Model file for the job. Use its own axes, mm. Coordinates: 2 decimals unless noted, no trailing zeros. Write each loop counter-clockwise with the first axis right and the second up, starting at its lowest first coordinate (ties: lowest second). Pieces come first, ordered by that corner, then holes. Notation, with made-up numbers: (62, 26.25) -> (85, 26.25) arc R10 ccw to (85, 44.25) -> close; hole circle Ø4 at (68.5, -35). An arc over 180 degrees is marked (long way). Answer as a JSON object with one key per item and string values. Group by question number.
Autodesk Inventor part; units mm, degrees
ref_plane "YZ Plane" through (0, 0, 0) normal (1, 0, 0) x (0, 1, 0)
ref_plane "XZ Plane" through (0, 0, 0) normal (0, 1, 0) x (-1, 0, 0)
ref_plane "XY Plane" through (0, 0, 0) normal (0, 0, 1) x (1, 0, 0)
sketch "main" plane through (0, 0, 0) normal (0, 0, 1) x (1, 0, 0)
  circle A0 centre (4.313, -2.5933) radius 2.0828
  circle A1 centre (17.2471, 11.4133) radius 2.1844
  circle A2 centre (-8.1529, 11.4133) radius 2.1844
  arc A3 (-8.1529, 16.1758) -> (-11.7104, 8.2471) centre (-8.1529, 11.4133) ccw
  arc A4 (20.746, 8.1824) -> (17.2471, 16.1758) centre (17.2471, 11.4133) ccw
  arc A5 (0.7554, -5.7596) -> (7.8119, -5.8243) centre (4.313, -2.5933) ccw
  line L0 (20.746, 8.1824) -> (7.8119, -5.8243)
  line L1 (17.2471, 16.1758) -> (-8.1529, 16.1758)
  line L2 (-11.7104, 8.2471) -> (0.7554, -5.7596)
  point P0 (4.4691, 6.7444)
  dimension "d0" = 4.1656
  dimension "d1" = 9.525
  dimension "d2" = 9.525
  dimension "d3" = 9.525
sketch "Sketch1" plane through (0, 0, 0) normal (0, 0, 1) x (1, 0, 0)
  circle A0 centre (-12.5245, 13.9543) radius 2.0828
  circle A1 centre (-25.3998, -0.1065) radius 2.1844
  circle A2 centre (0, 0) radius 2.1844
  arc A3 (0.02, -4.7625) -> (3.5443, 3.1811) centre (0, 0) ccw
  arc A4 (-28.9122, 3.1098) -> (-25.3798, -4.8689) centre (-25.3998, -0.1065) ccw
  arc A5 (-8.9802, 17.1354) -> (-16.0369, 17.1706) centre (-12.5245, 13.9543) ccw
  line L0 (-28.9122, 3.1098) -> (-16.0369, 17.1706)
  line L1 (-25.3798, -4.8689) -> (0.02, -4.7625)
  line L2 (3.5443, 3.1811) -> (-8.9802, 17.1354)
  point P0 (0, 0)
extrude "Extrusion1" add sketch "Sketch1" along normal blind 1.5875
properties part number "brace_gusset" material "Acetal Resin, White"
(1) Wall check: probe 1 along Y at (x, z) = (1, 0.5); probe 2 along X at (y, z) = (15.25, 0.75); probe 3 along Y at (x, z) = (-12, 0.85). Give the ranges that are in metal, low to high.
(2) Cut at A-A on x = -27. List the corners of the cut face in (y, z).
(3) Cut at B-B on y = 14.75. List the corners of the cut face in (x, z), plus the area to 3 significant figures.
(4) Cut at D-D on y = 8.5. List the corners of the cut face in (x, z).
(5) Cut at C-C on z = 0.7. List the corners of the cut face in (x, y), plus the area to 3 significant figures.
(6) Pin check, flat tips, straight feed: pin 1 (2.5 mm diameter, centred on x = -25.4, y = -0.11, fed in from +Z); pin 2 (10 mm diameter, centred on x = -21, y = 13.5, fed in from +Z). Stop position of each tip, or through.
(7) Pull direction X, two halves, no side cores. Call faces 1 (the face through (-12.556, 18.717, 0.783)), 2 (the face through (-27.133, 1.223, 0.783)), 3 (the face through (-13, 4, 0)): released by +X, released by -X, zero draft, split by the parting line, or undercut.
Results found:
{
 "1": {"probe 1": "y = -4.66 to -1.94, 1.94 to 6.02", "probe 2": "x = -17.8 to -14.16, -10.89 to -7.29", "probe 3": "y = -4.81 to 11.94, 15.97 to 18.69"},
 "2": {"outline": "(-4.59, 0) -> (-1.59, 0) -> (-1.59, 1.59) -> (-4.59, 1.59) -> close; (1.38, 0) -> (5.2, 0) -> (5.2, 1.59) -> (1.38, 1.59) -> close"},
 "3": {"outline": "(-18.25, 0) -> (-14.45, 0) -> (-14.45, 1.59) -> (-18.25, 1.59) -> close; (-10.6, 0) -> (-6.84, 0) -> (-6.84, 1.59) -> (-10.6, 1.59) -> close", "area": "12.0 mm²"},
 "4": {"outline": "(-23.98, 0) -> (-1.23, 0) -> (-1.23, 1.59) -> (-23.98, 1.59) -> close"},
 "5": {"outline": "(-28.91, 3.11) arc R4.76 ccw to (-25.38, -4.87) -> (0.02, -4.76) arc R4.76 ccw to (3.54, 3.18) -> (-8.98, 17.14) arc R4.76 ccw to (-16.04, 17.17) -> close; hole circle Ø4.37 at (-25.4, -0.11); hole circle Ø4.17 at (-12.52, 13.95); hole circle Ø4.37 at (0, 0)", "area": "507 mm²"},
 "6": {"pin 1": "passes through", "pin 2": "stops at z = 1.59"},
 "7": {"face 1": "split by the parting line", "face 2": "undercut", "face 3": "zero draft"}
}
